Verification items for the finished model (mm, model axes). A direction names the side the tool comes from. Give positions to 0.01 mm unless a question says otherwise; leave off trailing zeros. Order: outer loops, then holes, each group sorted by start corner. A loop starts at its lowest first (then second) coordinate and runs counter-clockwise, first axis right, second up.
from build123d import *

# Parameters (mm, degrees)
SKETCH1_R           = 1.65
BOSS_EXTRUDE1_DEPTH = 3
SKETCH2_W           = 69
SKETCH2_H           = 36.5
BOSS_EXTRUDE2_DEPTH = 4
BOSS_EXTRUDE3_DEPTH = 10
SKETCH4_W           = 75
SKETCH4_H           = 4.1
BOSS_EXTRUDE4_DEPTH = 6
SKETCH5_R           = 1.45
CUT_EXTRUDE1_DEPTH  = 93.2239123


with BuildPart() as part:
    # Sketch1 → Boss-Extrude1 (new body)
    with BuildSketch(Plane(origin=(0, 0, 0), x_dir=(1, 0, 0), z_dir=(0, 1, 0))):
        Polygon((-78, 39.5), (-78, 33.5), (-72, 33.5), (-72, 2), (-78, 2), (-78, -4), (9, -4), (9, 2), (3, 2), (3, 33.5), (9, 33.5), (9, 39.5), align=None)
        with Locations(Location((-75, 36.5, 0), (0, 0, 270))):
            Circle(SKETCH1_R, mode=Mode.SUBTRACT)
        with Locations(Location((6, 36.5, 0), (0, 0, 270))):
            Circle(SKETCH1_R, mode=Mode.SUBTRACT)
        with Locations(Location((-75, -1, 0), (0, 0, 270))):
            Circle(SKETCH1_R, mode=Mode.SUBTRACT)
        with Locations(Location((6, -1, 0), (0, 0, 270))):
            Circle(SKETCH1_R, mode=Mode.SUBTRACT)
    extrude(amount=BOSS_EXTRUDE1_DEPTH)

    # Sketch2 → Boss-Extrude2 (add)
    with BuildSketch(Plane(origin=(0, 3, 0), x_dir=(1, 0, 0), z_dir=(0, 1, 0))):
        Polygon((-72, 39.5), (-72, 33.5), (-72, 2), (-72, -4), (3, -4), (3, 2), (3, 33.5), (3, 39.5), align=None)
        with Locations((-34.5, 17.75)):
            Rectangle(SKETCH2_W, SKETCH2_H, mode=Mode.SUBTRACT)
    extrude(amount=BOSS_EXTRUDE2_DEPTH)

    # Sketch3 → Boss-Extrude3 (add)
    with BuildSketch(Plane(origin=(0, 7, 0), x_dir=(1, 0, 0), z_dir=(0, 1, 0))):
        Polygon((3, -4), (3, 0.1), (0, 0.1), (0, -0.5), (-7, -0.5), (-7, -4), align=None)
        Polygon((3, 39.5), (-7, 39.5), (-7, 36), (0, 36), (0, 35.4), (3, 35.4), align=None)
        Polygon((-72, 39.5), (-72, 35.4), (-69, 35.4), (-69, 36), (-62, 36), (-62, 39.5), align=None)
        Polygon((-72, -4), (-62, -4), (-62, -0.5), (-69, -0.5), (-69, 0.1), (-72, 0.1), align=None)
    extrude(amount=BOSS_EXTRUDE3_DEPTH)

    # Sketch4 → Boss-Extrude4 (add)
    with BuildSketch(Plane(origin=(0, 17, 0), x_dir=(1, 0, 0), z_dir=(0, 1, 0))):
        with Locations((-34.5, 37.45)):
            Rectangle(SKETCH4_W, SKETCH4_H)
        with Locations((-34.5, -1.95)):
            Rectangle(SKETCH4_W, SKETCH4_H)
    extrude(amount=BOSS_EXTRUDE4_DEPTH)

    # Sketch5 → Cut-Extrude1 (cut, through all)
    with BuildSketch(Plane.XY.offset(4)):
        with Locations((-68, 20)):
            Circle(SKETCH5_R)
        with Locations((-45.666666667, 20)):
            Circle(SKETCH5_R)
        with Locations((-23.333333333, 20)):
            Circle(SKETCH5_R)
        with Locations((-1, 20)):
            Circle(SKETCH5_R)
    extrude(amount=-CUT_EXTRUDE1_DEPTH, mode=Mode.SUBTRACT)


solid = part.part
(1) Set-up check for faces 1 (the flat face through (0, 5, -19)), 2 (the flat face through (-71, 7, -18)), 3 (the flat face through (5, 3, -35)), 4 (the flat face through (-62, 12, -38)), 5 (the flat face through (-73.7, 3, -0.4)): record each of +Z, -Z, +X, -X, +Y, -Y from which the full face is reachable in a straight line by a thin tool's end or side.
Solved:
face 1: none
face 2: +X, -X, +Y
face 3: +Z, -Z, +X, +Y
face 4: +Z, -Z
face 5: +Z, -Z, -X, +Y
(2) Scan lines: line 1 (Z direction, x = -34.5, y = 17.25); line 2 (X direction, y = 3.75, z = -19.5); line 3 (Y direction, x = -1, z = -36.6). Record each from-to range of solid material in increasing order.
Solved:
line 1: z = -39.5 to -35.4, -0.1 to 4
line 2: x = -72 to -69, 0 to 3
line 3: y = 0 to 18.55, 21.45 to 23
(3) Section check B-B, the plane x = 6. Enter the section's corners in (y, z).
Solved:
outline: (0, -39.5) - (3, -39.5) - (3, -38.15) - (0, -38.15) - close; (0, -34.85) - (3, -34.85) - (3, -33.5) - (0, -33.5) - close; (0, -2) - (3, -2) - (3, -0.65) - (0, -0.65) - close; (0, 2.65) - (3, 2.65) - (3, 4) - (0, 4) - close
(4) Section check C-C, the plane y = 13.25. Enter the section's corners in (x, z), then the cut area to 3 significant figures.
Solved:
outline: (-72, -39.5) - (-62, -39.5) - (-62, -36) - (-69, -36) - (-69, -35.4) - (-72, -35.4) - close; (-72, -0.1) - (-69, -0.1) - (-69, 0.5) - (-62, 0.5) - (-62, 4) - (-72, 4) - close; (-7, -39.5) - (3, -39.5) - (3, -35.4) - (0, -35.4) - (0, -36) - (-7, -36) - close; (-7, 0.5) - (0, 0.5) - (0, -0.1) - (3, -0.1) - (3, 4) - (-7, 4) - close
area: 147 mm2
(5) Section check D-D, the plane y = 5. Enter the section's corners in (x, z), then the cut area to 3 significant figures.
Solved:
outline: (-72, -39.5) - (3, -39.5) - (3, 4) - (-72, 4) - close; hole (-69, -36) - (0, -36) - (0, 0.5) - (-69, 0.5) - close
area: 744 mm2
(6) Go/stop test with flat-tipped pins: pin 1 (2 mm diameter, centred on y = 3, z = -11.5, fed in from +X); pin 2 (1.5 mm diameter, centred on y = 8, z = -30, fed in from -X); pin 3 (5 mm diameter, centred on x = -75, z = 0.5, fed in from +Y); pin 4 (8 mm diameter, centred on x = -65.5, z = -10, fed in from +Y). Record where each tip stops, or that it passes through.
Solved:
pin 1: stops at x = 3
pin 2: passes through
pin 3: stops at y = 3
pin 4: stops at y = 7
(7) Section check A-A, the plane x = -49.5. Enter the section's corners in (y, z), then the cut area to 3 significant figures.
Solved:
outline: (0, -39.5) - (7, -39.5) - (7, -36) - (3, -36) - (3, 0.5) - (7, 0.5) - (7, 4) - (0, 4) - close; (17, -39.5) - (23, -39.5) - (23, -35.4) - (17, -35.4) - close; (17, -0.1) - (23, -0.1) - (23, 4) - (17, 4) - close
area: 208 mm2
(8) Release check for a two-part mould opening along Z. For faces 6 (the flat face through (-35, 6, -39.5)), 7 (the cylindrical face through (-69.15, 19.12, -37.42)), 8 (the cylindrical face through (6.07, 1.48, -38.15)), 9 (the flat face through (3, 6, -17)) record: pulls with the +Z half, pulls with the -Z half, needs draft (parallel to the pull), parting line crosses it, or undercut.
Solved:
face 6: pulls with the -Z half
face 7: needs draft
face 8: undercut
face 9: undercut
